Geometry check sheet. Reference: drawing and pictorial views, mm from the part's lowest x, y, z. A direction names the side the tool comes from. Give positions to 0.01 mm unless a question says otherwise; leave off trailing zeros. Write each loop counter-clockwise with the first axis right and the second up, starting at its lowest first coordinate (ties: lowest second). Pieces come first, ordered by that corner, then holes. Notation, with made-up numbers: M 16.25,51 L 23.25,51 A30 cw 23.25,87 Z; hole C 41.25,6 d7. An arc over 180 degrees is marked long. Write item = value, one per line. Start each with the question number.
1) Scan lines: line 1 along Y through (x, z) = (12.25, 4); line 2 along Z through (x, y) = (16.25, 18.25). Record each from-to range of solid material in increasing order. Write a range as [from, to].
2) Go/stop test with flat-tipped pins: pin 1 (1.5 mm diameter, centred on y = 4, z = 4, fed in from +X); pin 2 (8 mm diameter, centred on x = 7, y = 5, fed in from +Z); pin 3 (6 mm diameter, centred on x = 2.5, z = 5, fed in from +Y). Record where each tip stops, or that it passes through.
3) Mould release check, pull along Y, two halves, no side actions. Record for the marked faces 1, 2 and 3: released by +Y, released by -Y, zero draft, split by the parting line, or undercut.
4) Access from +Z, -Z, +X, -X, +Y, -Y to the whole of each face (thin tool, end or side, straight path). Record for the marked faces 4, 5 and 6.
5) Cross-section at A-A, the plane x = 9.5. Record the cut outline in (y, z), plus the area to 3 significant figures.
6) Cross-section at D-D, the plane y = 1.75. Record the cut outline in (x, z).
7) Cross-section at C-C, the plane z = 18.25. Record the cut outline in (x, y), plus the area to 3 significant figures.
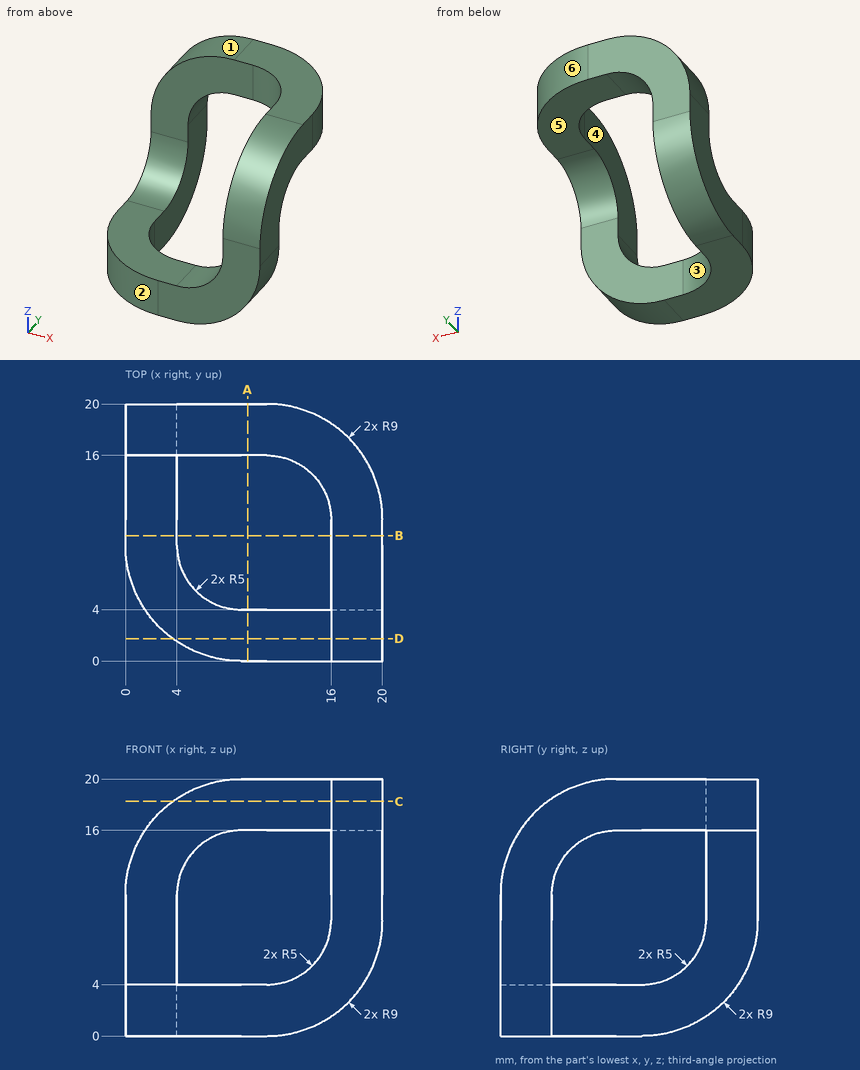
Reply:
q1.line_1 = [0, 4]
q1.line_2 = [16, 20]
q2.pin_1 = 18.93
q2.pin_2 = 4
q2.pin_3 = 19.94
q3.face_1 = zero draft
q3.face_2 = released by -Y
q3.face_3 = released by +Y
q4.face_4 = +Z, -X, -Y
q4.face_5 = -Z, +X, +Y
q4.face_6 = +Z, -Z, +X, +Y
q5.outline = M 0,0 L 4,0 L 4,4 L 0,4 Z; M 16,16 L 20,16 L 20,20 L 16,20 Z
q5.area = 32.0 mm2
q6.outline = M 3.67,0 L 11,0 A9 ccw 20,9 L 20,16.33 L 16,16.33 L 16,9 A5 cw 11,4 L 3.67,4 Z
q7.outline = M 3.67,16 L 11,16 A5 cw 16,11 L 16,3.67 L 20,3.67 L 20,11 A9 ccw 11,20 L 3.67,20 Z
q7.area = 103 mm2
